Input: part model. Units: mm. Frame: model coordinates. A direction names the side the tool comes from. Round coordinates to 2 decimals unless told otherwise and drop trailing zeros. Order: outer loops, then holes, each group sorted by start corner. A loop starts at its lowest first (then second) coordinate and runs counter-clockwise, first axis right, second up.
Item 1: Line query: L1, parallel to Z at x = 35, y = 13.5; L2, parallel to Z at x = -35, y = 13.5; L3, parallel to X at y = 10.75, z = 0. Output: solid intervals per line, ascending.
Item 2: Reachability of faces 5 (the cylindrical face through (41.6, 10.14, -26.64)), 6 (the flat face through (-15.511, 3.698, 7.368)), 7 (the cylindrical face through (37.385, 5.07, 19.249)), 8 (the flat face through (37, 10, -18)), 9 (the flat face through (-45, 10, -17.5)) from +Z, -Z, +X, -X, +Y, -Y: full face, straight path, thin tool, end or side. Return the list, or none.
Item 3: Mould query, pull axis X, two halves, no side actions, for faces 1 (the cylindrical face through (31, 15, -17)), 2 (the flat face through (-26.5, 4, -30)), 3 (the flat face through (-12, 10, -37)), 4 (the flat face through (-42.5, 10, 3)). Classes: released by +X, released by -X, zero draft, split by the parting line, or undercut.
Item 4: First-contact query: pin 1 (8 mm diameter, centred on x = -22, z = -25.5, fed in from -Y); pin 2 (1 mm diameter, centred on x = 16, y = 14, fed in from -Z); pin 3 (10 mm diameter, centred on x = 25, z = -33.5, fed in from +Y); pin 4 (12 mm diameter, centred on y = 7, z = 15.5, fed in from -X). Flat tips, straight axial feed; report the tip coordinate or a pass-through.
Item 5: Cut plane D-D on y = 13. Output: boundary loops of the cut face in (x, z), then the cut area to 3 significant figures.
Item 6: Cut plane A-A on z = -30. Output: boundary loops of the cut face in (x, y).
Item 7: Cut plane B-B on x = 3. Output: boundary loops of the cut face in (y, z).
Item 8: Cut plane C-C on z = 20. Output: boundary loops of the cut face in (x, y).
```python
from build123d import *

# Parameters (mm, degrees)
SALIENTE_EXTRUIR1_DEPTH = 20
CROQUIS2_R              = 2.5
CROQUIS2_R_2            = 5
CORTAR_EXTRUIR1_DEPTH   = 20
CROQUIS3_R              = 4
CROQUIS3_R_2            = 5
CORTAR_EXTRUIR2_DEPTH   = 20
CORTAR_EXTRUIR3_DEPTH   = 7.5
CROQUIS5_R              = 5
CROQUIS5_W              = 15
CROQUIS5_H              = 15
CORTAR_EXTRUIR4_DEPTH   = 10
REDONDEO1_R             = 3


with BuildPart() as part:
    # Croquis1 → Saliente-Extruir1 (new body)
    with BuildSketch(Plane(origin=(0, 0, 0), x_dir=(1, 0, 0), z_dir=(0, 1, 0))):
        Polygon((-2.5, 27.5), (-2.5, 42.5), (-47.5, 42.5), (-47.5, 17.5), (-42.5, 17.5), (-42.5, -27.5), (42.5, -27.5), (42.5, 27.5), align=None)
    extrude(amount=SALIENTE_EXTRUIR1_DEPTH)

    # Croquis2 → Cortar-Extruir1 (cut)
    with BuildSketch(Plane(origin=(0, 20, 0), x_dir=(1, 0, 0), z_dir=(0, 1, 0))):
        with Locations((35, 20)):
            Circle(CROQUIS2_R)
        with Locations((35, -20)):
            Circle(CROQUIS2_R)
        with Locations((-35, -20)):
            Circle(CROQUIS2_R)
        with Locations((-10, 35)):
            Circle(CROQUIS2_R)
        with Locations((-19.75, 0)):
            Circle(CROQUIS2_R_2)
        with Locations((19.75, 0)):
            Circle(CROQUIS2_R_2)
    extrude(amount=-CORTAR_EXTRUIR1_DEPTH, mode=Mode.SUBTRACT)

    # Croquis3 → Cortar-Extruir2 (cut)
    with BuildSketch(Plane(origin=(0, 20, 0), x_dir=(1, 0, 0), z_dir=(0, 1, 0))):
        with Locations((-35, 30)):
            Circle(CROQUIS3_R)
        with Locations((0, 17.5)):
            Circle(CROQUIS3_R_2)
    extrude(amount=-CORTAR_EXTRUIR2_DEPTH, mode=Mode.SUBTRACT)

    # Croquis4 → Cortar-Extruir3 (cut)
    with BuildSketch(Plane.XZ):
        Polygon((19.75, -9.814954576), (28.25, -4.907477288), (28.25, 4.907477288), (19.75, 9.814954576), (11.25, 4.907477288), (11.25, -4.907477288), align=None)
        Polygon((-19.655862416, -9.814503118), (-11.203322183, -4.82572602), (-11.297459766, 4.988777098), (-19.844137584, 9.814503118), (-28.296677817, 4.82572602), (-28.202540234, -4.988777098), align=None)
        Polygon((-35, -39.814954576), (-26.5, -34.907477288), (-26.5, -25.092522712), (-35, -20.185045424), (-43.5, -25.092522712), (-43.5, -34.907477288), align=None)
    extrude(amount=-CORTAR_EXTRUIR3_DEPTH, mode=Mode.SUBTRACT)

    # Croquis5 → Cortar-Extruir4 (cut)
    with BuildSketch(Plane(origin=(0, 20, 0), x_dir=(1, 0, 0), z_dir=(0, 1, 0))):
        with Locations((-35, -20)):
            Circle(CROQUIS5_R)
        with Locations((35, -20)):
            Circle(CROQUIS5_R)
        with Locations((35, 20)):
            Circle(CROQUIS5_R)
        with Locations((-10, 35)):
            Rectangle(CROQUIS5_W, CROQUIS5_H)
    extrude(amount=-CORTAR_EXTRUIR4_DEPTH, mode=Mode.SUBTRACT)

    # Redondeo1
    redondeo1_edges = [part.edges().sort_by_distance(p)[0] for p in [
        (-2.5, 5, -42.5),
        (42.5, 10, 27.5),
        (-42.5, 10, 27.5),
        (-47.5, 10, -42.5),
        (42.5, 10, -27.5),
    ]]
    fillet(redondeo1_edges, radius=REDONDEO1_R)


solid = part.part
```
From the geometry:
1. L1: z = -27.5 to -25, -15 to 15, 25 to 27.5
1. L2: z = -42.5 to -34, -26 to 15, 25 to 27.5
1. L3: x = -42.5 to -24.75, -14.75 to 14.75, 24.75 to 42.5
2. face 5: -Z, +X, +Y, -Y
2. face 6: -Y
2. face 7: +Y, -Y
2. face 8: +Y
2. face 9: +Z, -X, +Y, -Y
3. face 1: undercut
3. face 2: undercut
3. face 3: zero draft
3. face 4: released by -X
4. pin 1: stops at y = 0
4. pin 2: stops at z = -27.5
4. pin 3: passes through
4. pin 4: stops at x = -42.5
5. outline: (-47.5, -39.5) arc R3 ccw to (-44.5, -42.5) - (-17.5, -42.5) - (-17.5, -27.5) - (39.5, -27.5) arc R3 ccw to (42.5, -24.5) - (42.5, 24.5) arc R3 ccw to (39.5, 27.5) - (-39.5, 27.5) arc R3 ccw to (-42.5, 24.5) - (-42.5, -17.5) - (-47.5, -17.5) - close; hole circle Ø10 at (-35, 20); hole circle Ø8 at (-35, -30); hole circle Ø10 at (-19.75, 0); hole circle Ø10 at (0, -17.5); hole circle Ø10 at (19.75, 0); hole circle Ø10 at (35, -20); hole circle Ø10 at (35, 20)
5. area: 4,650 mm2
6. outline: (-47.5, 0) - (-43.5, 0) - (-43.5, 7.5) - (-39, 7.5) - (-39, 20) - (-47.5, 20) - close; (-31, 7.5) - (-26.5, 7.5) - (-26.5, 0) - (-2.5, 0) - (-2.5, 10) - (-17.5, 10) - (-17.5, 20) - (-31, 20) - close
7. outline: (0, -27.5) - (20, -27.5) - (20, -21.5) - (0, -21.5) - close; (0, -13.5) - (20, -13.5) - (20, 27.5) - (0, 27.5) - close
8. outline: (-42.5, 0) - (-37.5, 0) - (-37.5, 10) - (-40, 10) - (-40, 20) - (-42.5, 20) - close; (-32.5, 0) - (32.5, 0) - (32.5, 10) - (30, 10) - (30, 20) - (-30, 20) - (-30, 10) - (-32.5, 10) - close; (37.5, 0) - (42.5, 0) - (42.5, 20) - (40, 20) - (40, 10) - (37.5, 10) - close
